Model file for the job. Use its own axes, mm. Face numbers are marked on the shaded views. A direction names the side the tool comes from. Round coordinates to 2 decimals unless told otherwise and drop trailing zeros. Order: outer loops, then holes, each group sorted by start corner. A loop starts at its lowest first (then second) coordinate and runs counter-clockwise, first axis right, second up. Notation, with made-up numbers: (14.5, -18) -> (52.5, -18) arc R24 ccw to (52.5, 10) -> close; hole circle Ø5 at (30, 84.25). An arc over 180 degrees is marked (long way). Answer as CSV lines item,"result".
Autodesk Fusion 360 part; units mm, degrees
sketch "Sketch1" plane through (0, 0, 0) normal (1, 0, 0) x (0, 1, 0)
  line L0 (0, 0) -> (10, 0)
  line L1 (10, 0) -> (10, -18)
  line L2 (10, -18) -> (0, -18)
  line L3 (0, -18) -> (0, 0)
  line L4 (0, -18) -> (35, -18)
  line L5 (35, -18) -> (35, -15)
  line L6 (35, -15) -> (0, -15)
  line L7 (0, -15) -> (0, -18)
  line L8 (35, -18) -> (31, -18)
  line L9 (31, -18) -> (31, -6)
  line L10 (31, -6) -> (35, -6)
  line L11 (35, -6) -> (35, -18)
  line L12 (10, 0) -> (31, 0)
  line L13 (31, 0) -> (31, -15)
  line L14 (31, -15) -> (10, -15)
  line L15 (10, -15) -> (10, 0)
  line L16 (35, 0) -> (56, 0)
  line L17 (60, -6) -> (60, -18)
  line L18 (56, -6) -> (60, -6)
  line L19 (56, 0) -> (56, -15)
  line L20 (56, -18) -> (56, -6)
  line L21 (60, -18) -> (56, -18)
  line L22 (25, -18) -> (60, -18)
  line L23 (60, -15) -> (25, -15)
  line L24 (35, -15) -> (35, 0)
  line L25 (35, 0) -> (35, -18)
  line L26 (60, 0) -> (81, 0)
  line L27 (85, -6) -> (85, -18)
  line L28 (81, -6) -> (85, -6)
  line L29 (81, 0) -> (81, -15)
  line L30 (81, -18) -> (81, -6)
  line L31 (85, -18) -> (81, -18)
  line L32 (50, -18) -> (85, -18)
  line L33 (85, -15) -> (50, -15)
  line L34 (60, -15) -> (60, 0)
  line L35 (60, 0) -> (60, -18)
  line L36 (85, 0) -> (106, 0)
  line L37 (110, -6) -> (110, -18)
  line L38 (106, -6) -> (110, -6)
  line L39 (106, 0) -> (106, -15)
  line L40 (106, -18) -> (106, -6)
  line L41 (110, -18) -> (106, -18)
  line L42 (75, -18) -> (110, -18)
  line L43 (110, -15) -> (75, -15)
  line L44 (85, -15) -> (85, 0)
  line L45 (85, 0) -> (85, -18)
  line L46 (110, 0) -> (131, 0)
  line L47 (135, -6) -> (135, -18)
  line L48 (131, -6) -> (135, -6)
  line L49 (131, 0) -> (131, -15)
  line L50 (131, -18) -> (131, -6)
  line L51 (135, -18) -> (131, -18)
  line L52 (100, -18) -> (135, -18)
  line L53 (135, -15) -> (100, -15)
  line L54 (110, -15) -> (110, 0)
  line L55 (110, 0) -> (110, -18)
  line L56 (135, -18) -> (141, -18)
  line L57 (141, -18) -> (141, -14.9934)
  line L58 (141, -14.9934) -> (135, -14.9934)
  line L59 (135, -14.9934) -> (135, -18)
  line L60 (141, -18) -> (144, -18)
  line L61 (144, -18) -> (144, 0)
  line L62 (144, 0) -> (141, 0)
  line L63 (141, 0) -> (141, -18)
  dimension "d1" = 10
  dimension "d2" = 18
  dimension "d3" = 35
  dimension "d4" = 3
  dimension "d5" = 4
  dimension "d6" = 12
  dimension "d17" = 21
  dimension "d20" = 100
  dimension "d21" = 0
  dimension "d22" = 6
  dimension "d23" = 3
  dimension "d24" = 18
extrude "Extrude1" add sketch "Sketch1" along normal blind 22 contours L0 L1 L3 L6 L15 | L1 L2 L3 L4 L6 L7 | L1 L4 L6 L9 L14 L22 L23 | L6 L9 L10 L11 L13 L23 L24 L25 | L4 L5 L6 L8 L9 L11 L22 L23 L25 | L5 L11 L20 L22 L23 L25 L32 L33 | L17 L20 L21 L22 L23 L32 L33 L35 | L17 L18 L19 L20 L23 L33 L34 L35 | L17 L30 L32 L33 L35 L42 L43 | L27 L30 L31 L32 L33 L42 L43 L45 | L27 L28 L29 L30 L33 L43 L44 L45 | L27 L40 L42 L43 L45 L52 L53 | L37 L40 L41 L42 L43 L52 L53 L55 | L37 L38 L39 L40 L43 L53 L54 L55 | L37 L50 L52 L53 L55 | L47 L50 L51 L52 L53 L59 | L47 L48 L49 L50 L53 L59 | L47 L56 L57 L58 L59 L63 | L57 L60 L61 L62 L63
sketch "Sketch2" plane through (0, 0, 0) normal (0, -1, 0) x (1, 0, 0)
  line L0 (0, 0) -> (0, -18)
  line L1 (0, -18) -> (22, -18)
  line L2 (22, -18) -> (22, 0)
  line L3 (22, 0) -> (0, 0)
  line L4 (0, 0) -> (22.1644, 0)
  line L5 (22.1644, 0) -> (22.1644, -6)
  line L6 (22.1644, -6) -> (0, -6)
  line L7 (0, -6) -> (0, 0)
  circle A0 centre (11.0822, -6) radius 0.5
  dimension "d9" = 6
  dimension "d10" = 1
hole "Hole1" at (11.0822, 0, -6) direction (0, 1, 0) diameter 1.2 depth 136 tip angle 140
chamfer "Chamfer1" distance 4 angle 45 14 edges at (0, 5, 0) (22, 5, 0) (0, 33, -6) (22, 33, -6) (22, 58, -6) (0, 58, -6) (0, 83, -6) (22, 83, -6) (0, 108, -6) (0, 133, -6) (22, 133, -6) (22, 108, -6) (22, 142.5, 0) (0, 142.5, 0)
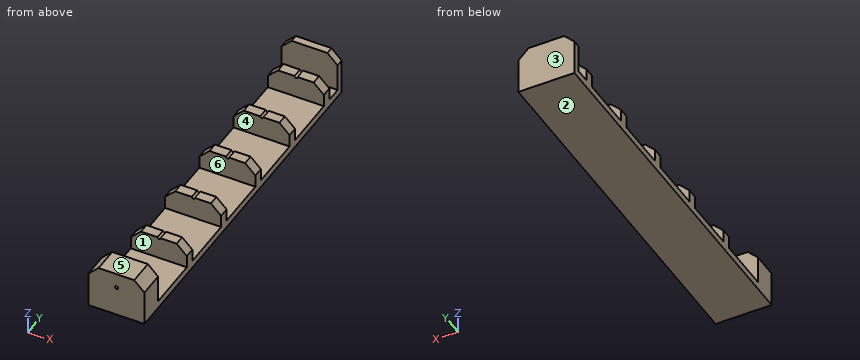
Q1. Saw through at C-C (x = 5.5). Write the cut outline in (y, z).
Checks:
outline,"(0, -18) -> (144, -18) -> (144, 0) -> (141, 0) -> (141, -14.99) -> (135, -14.99) -> (135, -6) -> (131, -6) -> (131, -15) -> (110, -15) -> (110, -6) -> (106, -6) -> (106, -15) -> (85, -15) -> (85, -6) -> (81, -6) -> (81, -15) -> (60, -15) -> (60, -6) -> (56, -6) -> (56, -15) -> (35, -15) -> (35, -6) -> (31, -6) -> (31, -15) -> (10, -15) -> (10, 0) -> (0, 0) -> close"
Q2. Wall check: L1, parallel to X at y = 3.5, z = -6; L2, parallel to Y at x = 12.25, z = -1.25; L3, parallel to Z at x = 11.5, y = 125.5. Give the ranges that are in metal, low to high. Write a range as [from, to].
Checks:
L1,"[0, 10.48], [11.68, 22]"
L2,"[0, 10], [141, 144]"
L3,"[-18, -15]"
Q3. Saw through at D-D (y = 23.5). Write the cut outline in (x, z), plus the area to 3 significant figures.
Checks:
outline,"(0, -18) -> (22, -18) -> (22, -15) -> (0, -15) -> close"
area,"66.0 mm²"
Q4. Tool access for the marked faces 1 and 2: list every direction of +Z, -Z, +X, -X, +Y, -Y with a clear straight run to the whole face (end or side of a thin tool).
Checks:
face 1,"+Z, +X, -X"
face 2,"-Z, +X, -X, +Y, -Y"
Q5. Flat gauge pins, fed straight in: pin 1 (1.2 mm diameter, centred on x = 8, y = 58.5, fed in from +Z); pin 2 (8 mm diameter, centred on x = 8.5, y = 116.5, fed in from +Z). Where does each tip first touch, or does it go through?
Checks:
pin 1,"z = -6"
pin 2,"z = -15"
Q6. Mould opens along Y. For the marked faces 3, 4, 5 and 6 say: +Y half, -Y half, draft (parallel to the pull), parting line (faces both ways), or undercut.
Checks:
face 3,"+Y half"
face 4,"undercut"
face 5,"draft"
face 6,"undercut"
Q7. Saw through at A-A (z = -11.75). Write the cut outline in (x, y), plus the area to 3 significant figures.
Checks:
outline,"(0, 0) -> (22, 0) -> (22, 10) -> (0, 10) -> close; (0, 31) -> (22, 31) -> (22, 35) -> (0, 35) -> close; (0, 56) -> (22, 56) -> (22, 60) -> (0, 60) -> close; (0, 81) -> (22, 81) -> (22, 85) -> (0, 85) -> close; (0, 106) -> (22, 106) -> (22, 110) -> (0, 110) -> close; (0, 131) -> (22, 131) -> (22, 135) -> (0, 135) -> close; (0, 141) -> (22, 141) -> (22, 144) -> (0, 144) -> close"
area,"726 mm²"
Q8. Saw through at B-B (x = 19.5). Write the cut outline in (y, z), plus the area to 3 significant figures.
Checks:
outline,"(0, -18) -> (144, -18) -> (144, -1.5) -> (141, -1.5) -> (141, -14.99) -> (135, -14.99) -> (135, -7.5) -> (131, -7.5) -> (131, -15) -> (110, -15) -> (110, -7.5) -> (106, -7.5) -> (106, -15) -> (85, -15) -> (85, -7.5) -> (81, -7.5) -> (81, -15) -> (60, -15) -> (60, -7.5) -> (56, -7.5) -> (56, -15) -> (35, -15) -> (35, -7.5) -> (31, -7.5) -> (31, -15) -> (10, -15) -> (10, -1.5) -> (0, -1.5) -> close"
area,"758 mm²"
